from build123d import *

# Parameters (mm, degrees)
BOSS_EXTRUDE1_DEPTH = 7.62
BOSS_EXTRUDE2_DEPTH = 6.004598
SKETCH12_R          = 2.1
SKETCH12_R_2        = 1.1
BOSS_EXTRUDE5_DEPTH = 6.0045981
SKETCH13_R          = 1.1
CUT_EXTRUDE5_DEPTH  = 6.0045981
SKETCH11_W          = 50
SKETCH11_H          = 1.6154019
CUT_EXTRUDE6_DEPTH  = 2
CUT_EXTRUDE7_DEPTH  = 4.0045981


with BuildPart() as part:
    # Sketch3 → Boss-Extrude1 (new body)
    with BuildSketch(Plane.XY):
        with BuildLine():
            Line((251.999999934, 224.000364601), (252, 159.907096774))
            Line((252, 159.907096774), (198, 159.907096774))
            Line((198, 159.907096774), (198.000000066, 247.000364601))
            ThreePointArc((198.000000066, 247.000364601), (199.464786475, 250.535213525), (202.999635399, 251.999999934))
            Line((202.999635399, 251.999999934), (224.416364601, 251.999999934))
            ThreePointArc((224.416364601, 251.999999934), (227.951213525, 250.535213525), (229.415999934, 247.000364601))
            Line((229.415999934, 247.000364601), (229.415999934, 230.000364601))
            ThreePointArc((229.415999934, 230.000364601), (229.709213468, 229.293213468), (230.416364601, 228.999999934))
            Line((230.416364601, 228.999999934), (247.000364601, 228.999999934))
            ThreePointArc((247.000364601, 228.999999934), (250.535213525, 227.535213525), (251.999999934, 224.000364601))
        make_face()
        with BuildLine():
            Line((200, 161.907096774), (250, 161.907096774))
            Line((250, 161.907096774), (250, 224))
            ThreePointArc((250, 224), (249.121, 226.121), (247, 227))
            Line((247, 227), (230.416, 227))
            ThreePointArc((230.416, 227), (228.295, 227.879), (227.416, 230))
            Line((227.416, 230), (227.416, 247))
            ThreePointArc((227.416, 247), (226.537, 249.121), (224.416, 250))
            Line((224.416, 250), (203, 250))
            ThreePointArc((203, 250), (200.879, 249.121), (200, 247))
            Line((200, 247), (200, 161.907096774))
        make_face(mode=Mode.SUBTRACT)
    extrude(amount=-BOSS_EXTRUDE1_DEPTH)



with BuildPart() as body_2:
    # Sketch5 → Boss-Extrude2 (new body)
    with BuildSketch(Plane(origin=(0, 0, -1.6154019), x_dir=(-1, 0, 0), z_dir=(0, 0, -1))):
        with BuildLine():
            Line((-200, 161.907096774), (-250, 161.907096774))
            Line((-250, 161.907096774), (-250, 224))
            ThreePointArc((-250, 224), (-249.121, 226.121), (-247, 227))
            Line((-247, 227), (-230.416, 227))
            ThreePointArc((-230.416, 227), (-228.295, 227.879), (-227.416, 230))
            Line((-227.416, 230), (-227.416, 247))
            ThreePointArc((-227.416, 247), (-226.537, 249.121), (-224.416, 250))
            Line((-224.416, 250), (-203, 250))
            ThreePointArc((-203, 250), (-200.879, 249.121), (-200, 247))
            Line((-200, 247), (-200, 161.907096774))
        make_face()
    extrude(amount=BOSS_EXTRUDE2_DEPTH)


with BuildPart() as part_1:
    add(part.part)

    add(body_2.part)  # Boss-Extrude5 merges body 2
    # Sketch12 → Boss-Extrude5 (add)
    # profile 1 of 4: a face of its own
    with BuildSketch(Plane(origin=(0, 0, -1.6154019), x_dir=(-1, 0, 0), z_dir=(0, 0, -1))):
        with Locations((-245, 166)):
            Circle(SKETCH12_R)
        with Locations((-245, 166)):
            Circle(SKETCH12_R_2, mode=Mode.SUBTRACT)
    # profile 2 of 4: a face of its own
    with BuildSketch(Plane(origin=(0, 0, -1.6154019), x_dir=(-1, 0, 0), z_dir=(0, 0, -1))):
        with Locations((-205, 166)):
            Circle(SKETCH12_R)
        with Locations((-205, 166)):
            Circle(SKETCH12_R_2, mode=Mode.SUBTRACT)
    # profile 3 of 4: a face of its own
    with BuildSketch(Plane(origin=(0, 0, -1.6154019), x_dir=(-1, 0, 0), z_dir=(0, 0, -1))):
        with Locations((-225, 224)):
            Circle(SKETCH12_R)
        with Locations((-225, 224)):
            Circle(SKETCH12_R_2, mode=Mode.SUBTRACT)
    # profile 4 of 4: a face of its own
    with BuildSketch(Plane(origin=(0, 0, -1.6154019), x_dir=(-1, 0, 0), z_dir=(0, 0, -1))):
        with Locations((-205, 224)):
            Circle(SKETCH12_R)
        with Locations((-205, 224)):
            Circle(SKETCH12_R_2, mode=Mode.SUBTRACT)
    extrude(amount=BOSS_EXTRUDE5_DEPTH)

    # Sketch13 → Cut-Extrude5 (cut)
    with BuildSketch(Plane(origin=(0, 0, -1.6154019), x_dir=(-1, 0, 0), z_dir=(0, 0, -1))):
        with Locations(Location((-225, 224, 0), (0, 0, 180))):
            Circle(SKETCH13_R)
        with Locations(Location((-205, 224, 0), (0, 0, 180))):
            Circle(SKETCH13_R)
        with Locations(Location((-205, 166, 0), (0, 0, 180))):
            Circle(SKETCH13_R)
        with Locations(Location((-245, 166, 0), (0, 0, 180))):
            Circle(SKETCH13_R)
    extrude(amount=CUT_EXTRUDE5_DEPTH, mode=Mode.SUBTRACT)

    # Sketch11 → Cut-Extrude6 (cut)
    with BuildSketch(Plane.XZ.offset(-159.907096774)):
        with Locations((225, -0.80770095)):
            Rectangle(SKETCH11_W, SKETCH11_H)
    extrude(amount=-CUT_EXTRUDE6_DEPTH, mode=Mode.SUBTRACT)

    # Sketch9 → Cut-Extrude7 (cut)
    with BuildSketch(Plane.XY.offset(-1.6154019)):
        with BuildLine():
            Line((200, 161.907096774), (250, 161.907096774))
            Line((250, 161.907096774), (250, 224))
            ThreePointArc((250, 224), (249.121, 226.121), (247, 227))
            Line((247, 227), (230.416, 227))
            ThreePointArc((230.416, 227), (228.295, 227.879), (227.416, 230))
            Line((227.416, 230), (227.416, 247))
            ThreePointArc((227.416, 247), (226.537, 249.121), (224.416, 250))
            Line((224.416, 250), (203, 250))
            ThreePointArc((203, 250), (200.879, 249.121), (200, 247))
            Line((200, 247), (200, 161.907096774))
        make_face()
    extrude(amount=-CUT_EXTRUDE7_DEPTH, mode=Mode.SUBTRACT)


solid = part_1.part
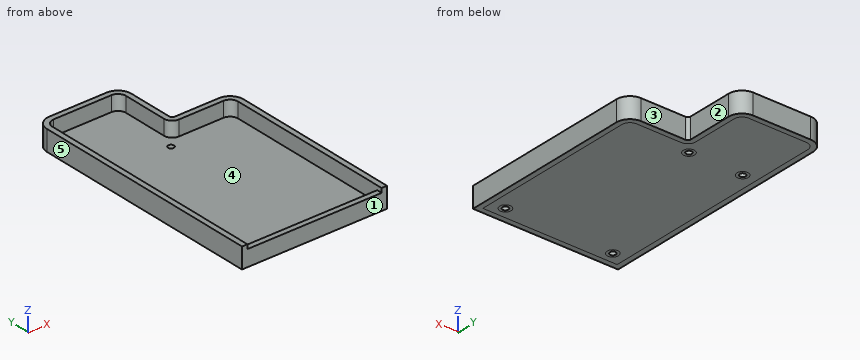
For this review, take the finished solid that the model builds, in its own axes (mm). Face numbers are marked on the shaded views. A direction names the side the tool comes from. Coordinates: 2 decimals unless noted, no trailing zeros. Write each loop counter-clockwise with the first axis right and the second up, starting at its lowest first coordinate (ties: lowest second). Pieces come first, ordered by that corner, then holes. Notation, with made-up numbers: (25, -10.5) -> (68, -10.5) arc R4 cw to (68, -4.5) -> close; hole circle Ø11 at (56, 88). An arc over 180 degrees is marked (long way). Write each question's results on one line, items separated by ' | '. Start each with the question number.
1) The part is to be moulded in two halves that separate along Y. For the marked faces 3, 4 and 5, say which applies: +Y half, -Y half, draft (parallel to the pull), parting line (faces both ways), or undercut.
2) Insertion check: pin 1 (2 mm diameter, centred on x = 205, y = 166, fed in from +Z); pin 2 (1.7 mm diameter, centred on x = 213.5, z = -1.5, fed in from -Y); pin 3 (3 mm diameter, centred on x = 236.5, y = 171.5, fed in from +Z); pin 4 (1.5 mm diameter, centred on x = 242.5, z = -5.5, fed in from +Y). Each pin has a flat end and moves straight along its axis. Give the tip position at first contact, or say it passes through.
3) Consider section D-D (x = 245). Write out the cut boundary in (y, z), plus the area to 3 significant figures.
4) Wall thickness on L1, parallel to X at y = 166, z = -6.45; L2, parallel to X at y = 219, z = -2; L3, parallel to Y at x = 205, z = -6.25: over which ranges is each line inside the solid? List them lowest first. Write a range as [from, to].
5) Consider section B-B (z = -3.75). Write out the cut boundary in (x, y).
6) Consider section C-C (y = 176.5). Write out the cut boundary in (x, z).
7) Consider section A-A (x = 205). Write out the cut boundary in (y, z).
8) For the marked faces 1 and 2, list the 3-axis set-ups (+Z, -Z, +X, -X, +Y, -Y) from which the entire face can be reached by the end or side of a thin tool; tool diameter is ignored.
Geometry says:
1) face 3: +Y half | face 4: undercut | face 5: draft
2) pin 1: through | pin 2: y = 159.91 | pin 3: z = -5.62 | pin 4: y = 229
3) outline: (159.91, -7.62) -> (164.9, -7.62) -> (164.9, -5.62) -> (161.91, -5.62) -> (161.91, -1.62) -> (159.91, -1.62) -> close; (167.1, -7.62) -> (229, -7.62) -> (229, 0) -> (227, 0) -> (227, -5.62) -> (167.1, -5.62) -> close | area: 153 mm^2
4) L1: [198, 203.9], [206.1, 243.9], [246.1, 252] | L2: [198, 200], [250, 252] | L3: [159.91, 164.9], [167.1, 222.9], [225.1, 252]
5) outline: (198, 159.91) -> (252, 159.91) -> (252, 224) arc R5 ccw to (247, 229) -> (230.42, 229) arc R1 cw to (229.42, 230) -> (229.42, 247) arc R5 ccw to (224.42, 252) -> (203, 252) arc R5 ccw to (198, 247) -> close; hole (200, 161.91) -> (250, 161.91) -> (250, 224) arc R3 ccw to (247, 227) -> (230.42, 227) arc R3 cw to (227.42, 230) -> (227.42, 247) arc R3 ccw to (224.42, 250) -> (203, 250) arc R3 ccw to (200, 247) -> close
6) outline: (198, -7.62) -> (252, -7.62) -> (252, 0) -> (250, 0) -> (250, -5.62) -> (200, -5.62) -> (200, 0) -> (198, 0) -> close
7) outline: (159.91, -7.62) -> (164.9, -7.62) -> (164.9, -5.62) -> (161.91, -5.62) -> (161.91, -1.62) -> (159.91, -1.62) -> close; (167.1, -7.62) -> (222.9, -7.62) -> (222.9, -5.62) -> (167.1, -5.62) -> close; (225.1, -7.62) -> (252, -7.62) -> (252, 0) -> (250, 0) -> (250, -5.62) -> (225.1, -5.62) -> close
8) face 1: +Z, -Z, +X, -X, -Y | face 2: +Z, -Z, +X, +Y
